The model under review builds one solid part; all positions refer to its coordinate system, in mm. Face numbers are marked on the shaded views. A direction names the side the tool comes from. Round coordinates to 2 decimals unless told otherwise and drop trailing zeros. Order: outer loops, then holes, each group sorted by start corner. A loop starts at its lowest first (then second) coordinate and runs counter-clockwise, first axis right, second up. Notation, with made-up numbers: M 34,82.25 L 54,82.25 A11 cw 54,86.25 Z; hole C -22.75,-22.75 d2. An arc over 180 degrees is marked long. Answer as CSV lines item,"result". Start each with the question number.
from build123d import *

# Parameters (mm, degrees)
F0_W          = 50
F0_H          = 30
F1_DEPTH      = 25
F1_DEPTH_BACK = 25
F2_W          = 45
F2_H          = 26
F3_DEPTH      = 47.5
F4_R          = 20.05
F5_DEPTH      = 3
F6_R          = 1.5
F7_DEPTH      = 1
F8_R          = 0.99999
F9_R          = 1


# Not quite as in the source:
# - a fillet or chamfer is up to 0.001 mm smaller than in the source, because OpenCascade refuses the exact size


with BuildPart() as f1:
    # F0 (on Front) → F1 (new body, two sides)
    with BuildSketch(Plane.XZ) as f1_sk:
        Rectangle(F0_W, F0_H)
    extrude(amount=F1_DEPTH)
    extrude(f1_sk.sketch, amount=-F1_DEPTH_BACK)

    # F2 (on face) → F3 (cut)
    with BuildSketch(Plane.XZ.offset(25)):
        with Locations((0, -2)):
            Rectangle(F2_W, F2_H)
    extrude(amount=-F3_DEPTH, mode=Mode.SUBTRACT)

    # F4 (on face) → F5 (cut)
    with BuildSketch(Plane(origin=(0, 0, 11), x_dir=(1, 0, 0), z_dir=(0, 0, -1))):
        Circle(F4_R)
    extrude(amount=-F5_DEPTH, mode=Mode.SUBTRACT)

    # F6 (on face) → F7 (join)
    with BuildSketch(Plane.XY.offset(15)):
        with Locations((-20, 20)):
            Circle(F6_R)
        with Locations((20, 20)):
            Circle(F6_R)
        with Locations((20, -20)):
            Circle(F6_R)
        with Locations((-20, -20)):
            Circle(F6_R)
    extrude(amount=F7_DEPTH)

    # F8 (radius 1 in the source; OpenCascade refuses exactly that, so slightly less here)
    f8_edges = [f1.edges().sort_by_distance(p)[0] for p in [
        (-21.5, -20, 16),
        (18.5, -20, 16),
        (18.5, 20, 16),
        (-21.5, 20, 16),
    ]]
    fillet(f8_edges, radius=F8_R)

    # F9
    f9_edges = [f1.edges().sort_by_distance(p)[0] for p in [
        (0, -25, 15),
        (25, 0, 15),
        (-25, 0, 15),
        (0, 25, 15),
        (18.5, -20, 15),
        (-21.5, -20, 15),
        (18.5, 20, 15),
        (-21.5, 20, 15),
        (-25, -25, 0),
        (25, -25, 0),
        (23.75, -25, -15),
        (22.5, -25, -2),
        (0, -25, 11),
        (-22.5, -25, -2),
        (-23.75, -25, -15),
        (25, 25, 0),
        (25, 0, -15),
        (0, 25, -15),
        (-25, 25, 0),
        (-25, 0, -15),
    ]]
    fillet(f9_edges, radius=F9_R)


solid = f1.part
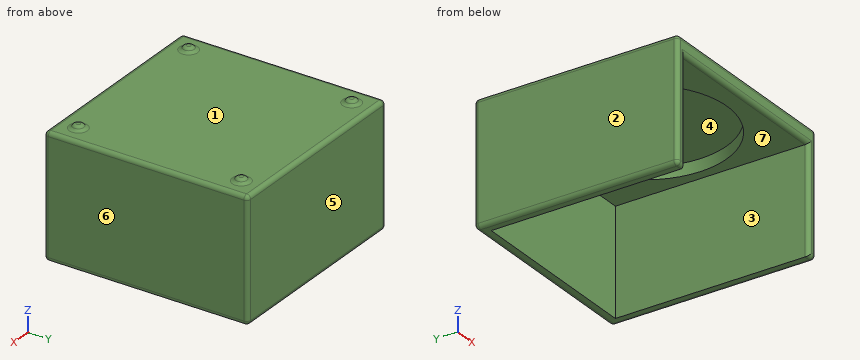
Item 1: The part is to be moulded in two halves that separate along X. For the marked faces 4, 5, 6 and 7, say which applies: +X half, -X half, draft (parallel to the pull), parting line (faces both ways), or undercut.
Item 2: For pin 1 (8 mm diameter, centred on x = -8.5, z = -8.5, fed in from -Y); pin 2 (12 mm diameter, centred on x = 9.5, y = 10.5, fed in from -Z); pin 3 (22.5 mm diameter, centred on x = -5, y = -3.5, fed in from -Z), all flat-tipped, find the tip position at first contact; note any pin that passes through.
Item 3: Wall thickness on probe 1 along X at (y, z) = (0, 12.35); probe 2 along X at (y, z) = (0, 2.5): over which ranges is each line inside the solid? List them lowest first. Write a range as [from, to].
Item 4: Consider section B-B (z = 2). State the section outline as (x, y) points, and give its area (3 significant figures).
Item 5: Consider section C-C (y = 0). State the section outline as (x, z) points, and give its area (3 significant figures).
Item 6: Tool access review of the marked faces 1, 2 and 3: name each direction out of +Z, -Z, +X, -X, +Y, -Y from which nothing blocks a thin tool from reaching the whole face with its end or side.
Item 7: Consider section D-D (y = 16.5). State the section outline as (x, z) points, and give its area (3 significant figures).
Item 8: Consider section A-A (x = 0). State the section outline as (y, z) points, and give its area (3 significant figures).
Reported:
1,face 4,"undercut"
1,face 5,"draft"
1,face 6,"+X half"
1,face 7,"undercut"
2,pin 1,"stops at y = 22.5"
2,pin 2,"stops at z = 11"
2,pin 3,"stops at z = 14"
3,probe 1,"x = [-25, -20.05], [20.05, 25]"
3,probe 2,"x = [-25, -22.5], [22.5, 25]"
4,outline,"M -25,-24 A1 ccw -24,-25 L -23.5,-25 A1 ccw -22.5,-24 L -22.5,22.5 L 22.5,22.5 L 22.5,-24 A1 ccw 23.5,-25 L 24,-25 A1 ccw 25,-24 L 25,24 A1 ccw 24,25 L -24,25 A1 ccw -25,24 Z"
4,area,"361 mm²"
5,outline,"M -25,-14 A1 ccw -24,-15 L -22.5,-15 L -22.5,11 L -20.05,11 L -20.05,14 L 20.05,14 L 20.05,11 L 22.5,11 L 22.5,-15 L 24,-15 A1 ccw 25,-14 L 25,14 A1 ccw 24,15 L -24,15 A1 ccw -25,14 Z"
5,area,"209 mm²"
6,face 1,"+Z"
6,face 2,"+Z, -Z, -X, +Y, -Y"
6,face 3,"-Z, -Y"
7,outline,"M -25,-14 A1 ccw -24,-15 L -22.5,-15 L -22.5,11 L -11.39,11 L -11.39,14 L 11.39,14 L 11.39,11 L 22.5,11 L 22.5,-15 L 24,-15 A1 ccw 25,-14 L 25,14 A1 ccw 24,15 L -24,15 A1 ccw -25,14 Z"
7,area,"261 mm²"
8,outline,"M -25,12 A1 ccw -24,11 L -20.05,11 L -20.05,14 L 20.05,14 L 20.05,11 L 22.5,11 L 22.5,-15 L 24,-15 A1 ccw 25,-14 L 25,14 A1 ccw 24,15 L -24,15 A1 ccw -25,14 Z"
8,area,"144 mm²"
